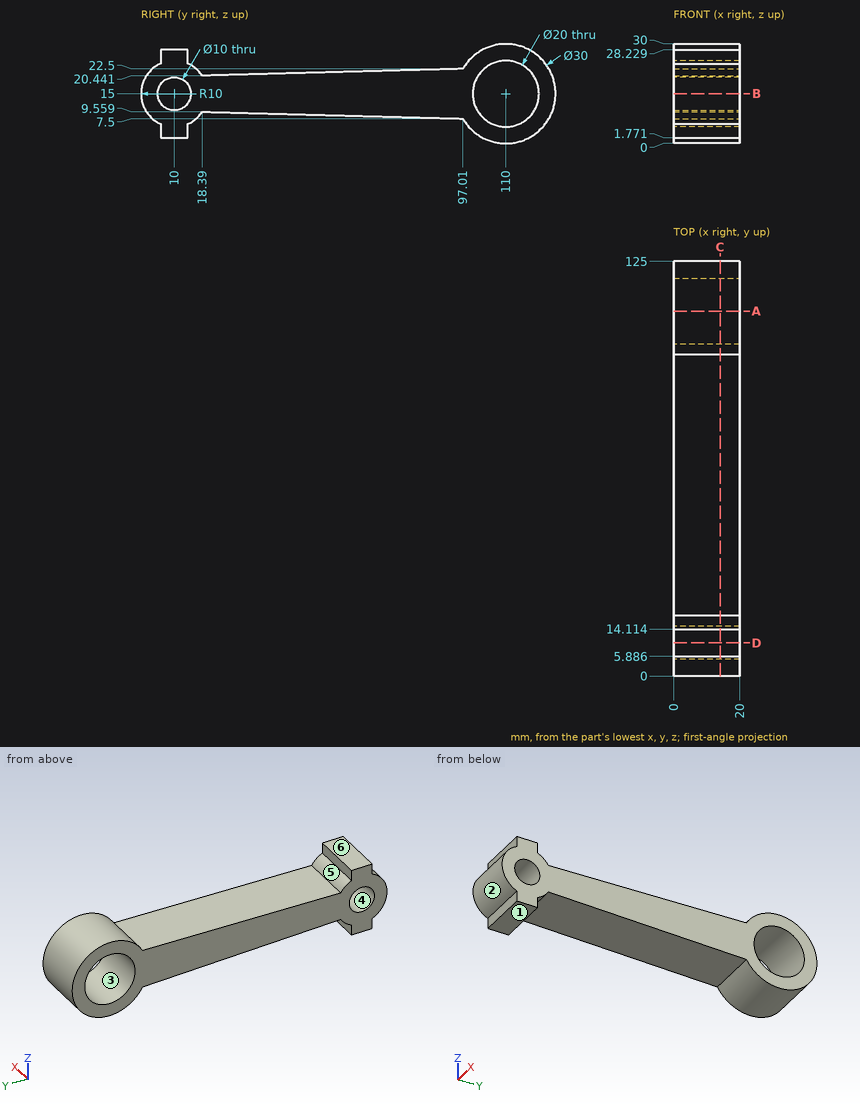
Study the drawing (mm; zero at the part's minimum x, y, z) and answer. A direction names the side the tool comes from. Give positions to 0.01 mm unless a question says otherwise; leave off trailing zeros. Loops run counter-clockwise (first coordinate to the right, second up) from the corner with the lowest first, then second, coordinate; pieces in that order, holes last. Notation, with made-up numbers: (78.5, 62.25) - (99.5, 62.25) arc R17 cw to (99.5, 81.25) - close; hole circle Ø3 at (85.25, 31.5). An arc over 180 degrees is marked (long way). Return JSON: item names as keys, results as strings. Group by question number.
1. Straight lines are drawn through the part: line 1 (Y direction, x = 10, z = 15); line 2 (Z direction, x = 11, y = 10); line 3 (Y direction, x = 4.25, z = 14.25). For each, find the intervals that lie inside material, in ascending order. Write a range as [from, to].
2. Given pin 1 Ø1 at (y, z) = (76, 6) entering from +X; pin 2 Ø6.5 at (x, y) = (11.5, 8) entering from +Z; pin 3 Ø4.5 at (x, z) = (7.5, 3.5) entering from -Y; pin 4 Ø1.5 at (x, y) = (16, 112) entering from +Z, each flat-ended and moving along its own axis, determine where each tip first touches the part or whether it passes through.
3. Find section C-C (x = 14). Write down the section's boundary in (y, z) (1 decimal).
4. Find section B-B (z = 15). Write down the section's boundary in (x, y).
5. Find section D-D (y = 10). Write down the section's boundary in (x, z), then the cut area to 3 significant figures.
6. Find section A-A (y = 110). Write down the section's boundary in (x, z), then the cut area to 3 significant figures.
7. Which of the six approach directions +Z, -Z, +X, -X, +Y, -Y give full straight-line access (tool end or side, diameter ignored) to the marked faces 4, 5 and 6?
8. Determine the mould class of the marked faces 1, 2 and 3 for opening direction Y: pulls with the +Y half, pulls with the -Y half, needs draft (parallel to the pull), parting line crosses it, or undercut.
Verdict:
{
 "1": {"line 1": "y = [0, 5], [15, 100], [120, 125]", "line 2": "z = [1.77, 10], [20, 28.23]", "line 3": "y = [0.03, 5.06], [14.94, 100.03], [119.97, 124.98]"},
 "2": {"pin 1": "passes through", "pin 2": "stops at z = 28.23", "pin 3": "stops at y = 5.89", "pin 4": "stops at z = 29.95"},
 "3": {"outline": "(5.9, 1.8) - (14.1, 1.8) - (14.1, 5.9) arc R10 ccw to (18.4, 9.6) - (97, 7.5) arc R15 ccw (long way) to (97, 22.5) - (18.4, 20.4) arc R10 ccw to (14.1, 24.1) - (14.1, 28.2) - (5.9, 28.2) - (5.9, 24.1) arc R10 ccw to (5.9, 5.9) - close; hole circle Ø10 at (10, 15); hole circle Ø20 at (110, 15)"},
 "4": {"outline": "(0, 0) - (20, 0) - (20, 5) - (0, 5) - close; (0, 15) - (20, 15) - (20, 100) - (0, 100) - close; (0, 120) - (20, 120) - (20, 125) - (0, 125) - close"},
 "5": {"outline": "(0, 1.77) - (20, 1.77) - (20, 10) - (0, 10) - close; (0, 20) - (20, 20) - (20, 28.23) - (0, 28.23) - close", "area": "329 mm^2"},
 "6": {"outline": "(0, 0) - (20, 0) - (20, 5) - (0, 5) - close; (0, 25) - (20, 25) - (20, 30) - (0, 30) - close", "area": "200 mm^2"},
 "7": {"face 4": "+X, -X", "face 5": "+Z, +X, -X", "face 6": "+Z, +X, -X, -Y"},
 "8": {"face 1": "needs draft", "face 2": "pulls with the -Y half", "face 3": "undercut"}
}
